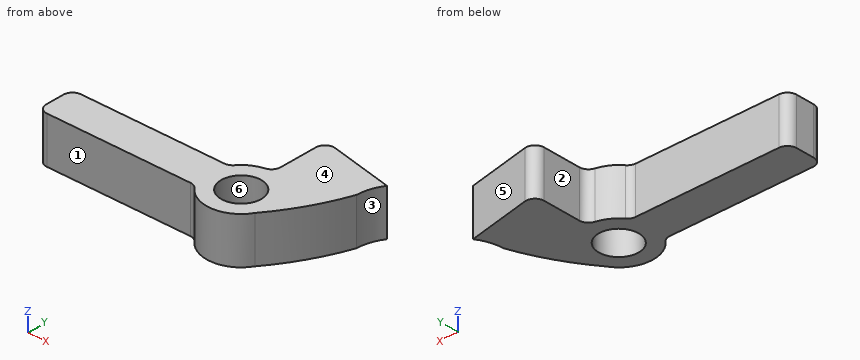
from build123d import *

# Parameters (mm, degrees)
SKETCH1_W           = 50
SKETCH1_H           = 50
BOSS_EXTRUDE1_DEPTH = 6.35
SKETCH2_OUTSIDE_W   = 66.2
SKETCH2_OUTSIDE_H   = 66.2
SKETCH2_OUTSIDE_R   = 2.75
CUT_EXTRUDE1_DEPTH  = 7.35


with BuildPart() as part:
    # Sketch1 → Boss-Extrude1 (new body)
    with BuildSketch(Plane.XY):
        with Locations((25, 25)):
            Rectangle(SKETCH1_W, SKETCH1_H)
    extrude(amount=BOSS_EXTRUDE1_DEPTH)

    # Sketch2 outside → Cut-Extrude1 (cut, through all)
    with BuildSketch(Plane(origin=(0, 0, 0), x_dir=(-1, 0, 0), z_dir=(0, 0, -1))):
        with Locations((-25, 25)):
            Rectangle(SKETCH2_OUTSIDE_W, SKETCH2_OUTSIDE_H)
        with BuildLine():
            Line((-26.850834583, 24.37770606), (-7.04230164, 24.37770606))
            ThreePointArc((-7.04230164, 24.37770606), (-6.144276028, 24.749680448), (-5.77230164, 25.64770606))
            Line((-5.77230164, 25.64770606), (-5.77230164, 28.18770606))
            ThreePointArc((-5.77230164, 28.18770606), (-6.144276028, 29.085731672), (-7.04230164, 29.45770606))
            Line((-7.04230164, 29.45770606), (-26.850834583, 29.45770606))
            ThreePointArc((-26.850834583, 29.45770606), (-27.395915456, 29.580628538), (-27.835480279, 29.925600797))
            ThreePointArc((-27.835480279, 29.925600797), (-29.039981102, 30.97869826), (-30.525270061, 31.573469818))
            ThreePointArc((-30.525270061, 31.573469818), (-31.245944628, 32.017090124), (-31.52790164, 32.81500682))
            Line((-31.52790164, 32.81500682), (-31.52790164, 38.057404626))
            ThreePointArc((-31.52790164, 38.057404626), (-31.996191822, 39.042372325), (-33.055714819, 39.300960963))
            Line((-33.055714819, 39.300960963), (-41.893380205, 37.485936348))
            ThreePointArc((-41.893380205, 37.485936348), (-41.111586239, 35.864517894), (-40.816192235, 34.08886534))
            ThreePointArc((-40.816192235, 34.08886534), (-38.634961437, 29.096054751), (-35.652347625, 24.53645606))
            ThreePointArc((-35.652347625, 24.53645606), (-31.908469933, 22.170435895), (-27.835480279, 23.909811323))
            ThreePointArc((-27.835480279, 23.909811323), (-27.395915456, 24.254783582), (-26.850834583, 24.37770606))
        make_face(mode=Mode.SUBTRACT)
        with Locations((-31.52790164, 26.91770606)):
            Circle(SKETCH2_OUTSIDE_R)
    extrude(amount=-CUT_EXTRUDE1_DEPTH, mode=Mode.SUBTRACT)


solid = part.part
Geometry check sheet. Reference: the model listing, model coordinates, mm. Face numbers are marked on the shaded views. A direction names the side the tool comes from. Give positions to 0.01 mm unless a question says otherwise; leave off trailing zeros. Loops run counter-clockwise (first coordinate to the right, second up) from the corner with the lowest first, then second, coordinate; pieces in that order, holes last. Notation, with made-up numbers: (43.25, 83) -> (80.25, 83) arc R22 ccw to (80.25, 99) -> close; hole circle Ø10 at (70.25, 51). An arc over 180 degrees is marked (long way). Answer in a Markdown table with one row per item. Add a question column.
1) Cross-section at A-A on x = 30. Record the boundary of the cut face in (y, z), and give its area (3 significant figures).
2) Gauge pin test, flat ends, axial feed: P1, Ø2, axis at y = 36, z = 1, coming from the +X side; P2, Ø1.9, axis at x = 17, z = 4, coming from the -Y side; P3, Ø3, axis at x = 17, z = 4, coming from the +Y side; P4, Ø4.5, axis at x = 31.53, y = 26.92, coming from the +Z side. Record the tip position at first contact, or that the pin passes through.
3) Set-up check for the marked faces 1, 2 and 3: record each of +Z, -Z, +X, -X, +Y, -Y from which the full face is reachable in a straight line by a thin tool's end or side.
4) Draft check along X on the marked faces 4, 5 and 6. Enter one of: pulls with the +X half, pulls with the -X half, needs draft (parallel to the pull), parting line crosses it, or undercut.
5) Material ranges on probe 1 along Y at (x, z) = (15.5, 6.25); probe 2 along X at (y, z) = (27.25, 2.5); probe 3 along X at (y, z) = (24.75, 5), recorded low to high. Write a range as from..to.
6) Cross-section at D-D on x = 20.5. Record the boundary of the cut face in (y, z), and give its area (3 significant figures).
7) Cross-section at B-B on y = 28.75. Record the boundary of the cut face in (x, z), and give its area (3 significant figures).
Outcome:
| question | item | result |
|---|---|---|
| 1 | outline | (22.41, 0) -> (24.63, 0) -> (24.63, 6.35) -> (22.41, 6.35) -> close; (29.2, 0) -> (31.43, 0) -> (31.43, 6.35) -> (29.2, 6.35) -> close |
| 1 | area | 28.2 mm^2 |
| 2 | P1 | stops at x = 41.6 |
| 2 | P2 | stops at y = 24.38 |
| 2 | P3 | stops at y = 29.46 |
| 2 | P4 | passes through |
| 3 | face 1 | +Z, -Z, -X, -Y |
| 3 | face 2 | +Z, -Z, -X, +Y |
| 3 | face 3 | +Z, -Z, +X, -Y |
| 4 | face 4 | needs draft |
| 4 | face 5 | pulls with the +X half |
| 4 | face 6 | undercut |
| 5 | probe 1 | y = 24.38..29.46 |
| 5 | probe 2 | x = 5.77..28.8, 34.26..37.56 |
| 5 | probe 3 | x = 6.14..29.84, 33.22..35.82 |
| 6 | outline | (24.38, 0) -> (29.46, 0) -> (29.46, 6.35) -> (24.38, 6.35) -> close |
| 6 | area | 32.3 mm^2 |
| 7 | outline | (5.9, 0) -> (29.48, 0) -> (29.48, 6.35) -> (5.9, 6.35) -> close; (33.58, 0) -> (38.45, 0) -> (38.45, 6.35) -> (33.58, 6.35) -> close |
| 7 | area | 181 mm^2 |
